Build history of the part. All positions in model axes, mm. A direction names the side the tool comes from. Round coordinates to 2 decimals unless told otherwise and drop trailing zeros. Order: outer loops, then holes, each group sorted by start corner. A loop starts at its lowest first (then second) coordinate and runs counter-clockwise, first axis right, second up. Notation, with made-up numbers: (81.5, 42.25) -> (126.5, 42.25) arc R20 cw to (126.5, 46.25) -> close; hole circle Ø7 at (5.25, 54.25). An arc over 180 degrees is marked (long way). Use a Markdown table: item, result. Add a question column.
Item 1: Pin check, flat tips, straight feed: pin 1 (10 mm diameter, centred on x = 21, z = 15, fed in from +Y); pin 2 (10 mm diameter, centred on x = 20.5, z = 15, fed in from -Y); pin 3 (3.5 mm diameter, centred on y = 40.5, z = 17, fed in from -X). Stop position of each tip, or through.
Item 2: Slice it at B-B, the plane x = 28.5. Give the cut face in (y, z), plus the area to 3 significant figures.
Item 3: Two-plate mould, pull along X, no slides. Class faces 6 (the face through (63.62, 37.564, 17.742)), 7 (the face through (20, 16, 8)), 8 (the face through (64.611, 10.115, 9.874)): released by +X, released by -X, zero draft, split by the parting line, or undercut.
Item 4: 3-axis set-ups, long thin cutter, end or side, ignore diameter. For faces 1 (the face through (65, 29.9, 10)), 2 (the face through (40.377, 17, 10)), 3 (the face through (20, 10, 4)), 4 (the face through (67.8, 55, 18)), 5 (the face through (55, 52, 10)): which of +Z, -Z, +X, -X, +Y, -Y reach the whole face in a straight line?
Item 5: Slice it at C-C, the plane z = 9.5. State how many separate pieces and enclosed holes the cut face has, plus the area to 3 significant figures.
Item 6: Slice it at A-A, the plane x = 5. Give the cut face in (y, z).
Item 7: Probe L1, parallel to X at y = 6.75, z = 10; L2, parallel to X at y = 6.5, z = 10; L3, parallel to X at y = 55, z = 3. List the from-to ranges inside material, lowest first.
from build123d import *

# Parameters (mm, degrees)
SKETCH_13_R          = 1.55
EXTRUDE_6_DEPTH      = 20
SKETCH_15_R          = 6.1
CUT_EXTRUDE_4_DEPTH  = 40.1
SKETCH_16_R          = 1.55
CUT_EXTRUDE_5_DEPTH  = 93.330926639
CUT_EXTRUDE_7_DEPTH  = 105.522724888
EXTRUDE_8_DEPTH      = 20
CUT_EXTRUDE_8_DEPTH  = 4
CUT_EXTRUDE_9_DEPTH  = 5
SKETCH_29_W          = 20
SKETCH_29_H          = 20
SKETCH_29_W_2        = 12
SKETCH_29_H_2        = 12
CUT_EXTRUDE_11_DEPTH = 40.376839
CHAMFER_7_SIZE       = 1


with BuildPart() as part:
    # 草图13 → 凸台-拉伸6 (new body)
    with BuildSketch(Plane.XY):
        Polygon((0, 0), (45, 0), (75, 0), (75, 70), (55, 70), (55, 20), (45, 20), (0, 20), align=None)
        with Locations((65, 40)):
            Circle(SKETCH_13_R, mode=Mode.SUBTRACT)
        with Locations((65, 55)):
            Circle(SKETCH_13_R, mode=Mode.SUBTRACT)
    extrude(amount=EXTRUDE_6_DEPTH)

    # 草图15 → 切除-拉伸4 (cut)
    with BuildSketch(Plane(origin=(0, 70, 0), x_dir=(1, 0, 0), z_dir=(0, 1, 0))):
        with Locations(Location((65, -10, 0), (0, 0, 270))):
            Circle(SKETCH_15_R)
    extrude(amount=-CUT_EXTRUDE_4_DEPTH, mode=Mode.SUBTRACT)

    # 草图16 → 切除-拉伸5 (cut, through all)
    with BuildSketch(Plane(origin=(0, 20, 0), x_dir=(1, 0, 0), z_dir=(0, 1, 0))):
        with Locations(Location((5, -10, 0), (0, 0, 270))):
            Circle(SKETCH_16_R)
        with Locations(Location((20, -10, 0), (0, 0, 270))):
            Circle(SKETCH_16_R)
        with Locations(Location((35, -10, 0), (0, 0, 270))):
            Circle(SKETCH_16_R)
    extrude(amount=-CUT_EXTRUDE_5_DEPTH, mode=Mode.SUBTRACT)

    # 草图24 → 切除-拉伸7 (cut, through all)
    with BuildSketch(Plane(origin=(0, 0, 0), x_dir=(-1, 0, 0), z_dir=(0, 0, -1))):
        with BuildLine():
            Line((-75, 35), (-75, 0))
            Line((-75, 0), (-40, 0))
            ThreePointArc((-40, 0), (-64.748737342, 10.251262658), (-75, 35))
        make_face()
    extrude(amount=-CUT_EXTRUDE_7_DEPTH, mode=Mode.SUBTRACT)

    # 草图25 → 凸台-拉伸8 (add)
    with BuildSketch(Plane(origin=(0, 0, 0), x_dir=(-1, 0, 0), z_dir=(0, 0, -1))):
        with BuildLine():
            Line((-55, 34.995265669), (-55, 20))
            Line((-55, 20), (-40.376838854, 20))
            ThreePointArc((-40.376838854, 20), (-50.739007934, 24.522744072), (-55, 34.995265669))
        make_face()
    extrude(amount=-EXTRUDE_8_DEPTH)

    # 草图26 → 切除-拉伸8 (cut)
    with BuildSketch(Plane.XZ):
        Polygon((4.044652328, 6.911206682), (7.197299644, 7.628247988), (8.152647316, 10.717041306), (5.955347672, 13.088793318), (2.802700356, 12.371752012), (1.847352684, 9.282958694), align=None)
        Polygon((19.044652328, 6.911206682), (22.197299644, 7.628247988), (23.152647316, 10.717041306), (20.955347672, 13.088793318), (17.802700356, 12.371752012), (16.847352684, 9.282958694), align=None)
        Polygon((34.044652328, 6.911206682), (37.197299644, 7.628247988), (38.152647316, 10.717041306), (35.955347672, 13.088793318), (32.802700356, 12.371752012), (31.847352684, 9.282958694), align=None)
    extrude(amount=-CUT_EXTRUDE_8_DEPTH, mode=Mode.SUBTRACT)

    # 草图27 → 切除-拉伸9 (cut)
    with BuildSketch(Plane(origin=(0, 0, 20), x_dir=(-1, 0, 0), z_dir=(0, 0, -1))):
        Polygon((-65, 36.766838493), (-62.2, 38.383419246), (-62.2, 41.616580754), (-65, 43.233161507), (-67.8, 41.616580754), (-67.8, 38.383419246), align=None)
        Polygon((-65, 51.766838493), (-62.2, 53.383419246), (-62.2, 56.616580754), (-65, 58.233161507), (-67.8, 56.616580754), (-67.8, 53.383419246), align=None)
    extrude(amount=CUT_EXTRUDE_9_DEPTH, mode=Mode.SUBTRACT)

    # 草图29 → 切除-拉伸11 (cut)
    with BuildSketch(Plane.ZY):
        with Locations((10, 10)):
            Rectangle(SKETCH_29_W, SKETCH_29_H)
        with Locations((10, 10)):
            Rectangle(SKETCH_29_W_2, SKETCH_29_H_2, mode=Mode.SUBTRACT)
    extrude(amount=-CUT_EXTRUDE_11_DEPTH, mode=Mode.SUBTRACT)

    # 倒角7
    chamfer_7_edges = [part.edges().sort_by_distance(p)[0] for p in [
        (55, 70, 10),
        (75, 70, 10),
        (65, 70, 20),
        (64.881613342, 10.384855932, 0),
        (64.881613342, 10.384855932, 20),
        (0, 16, 10),
        (20.1884195, 16, 16),
        (0, 4, 10),
        (20.1884195, 4, 4),
        (0, 10, 16),
        (20.1884195, 4, 16),
        (0, 10, 4),
        (20.1884195, 16, 4),
        (55, 52.497632834, 20),
        (65, 70, 3.9),
        (75, 52.5, 0),
        (75, 52.5, 20),
        (50.739007934, 24.522744072, 0),
        (50.739007934, 24.522744072, 20),
        (55, 52.497632834, 0),
        (65, 70, 0),
    ]]
    chamfer(chamfer_7_edges, length=CHAMFER_7_SIZE)


solid = part.part
Check sheet entries:
| question | item | result |
|---|---|---|
| 1 | pin 1 | y = 16 |
| 1 | pin 2 | y = 4 |
| 1 | pin 3 | x = 55 |
| 2 | outline | (4, 5) -> (5, 4) -> (15, 4) -> (16, 5) -> (16, 15) -> (15, 16) -> (5, 16) -> (4, 15) -> close |
| 2 | area | 142 mm2 |
| 3 | face 6 | undercut |
| 3 | face 7 | zero draft |
| 3 | face 8 | released by +X |
| 4 | face 1 | +Y |
| 4 | face 2 | -X |
| 4 | face 3 | -Z, -X, +Y, -Y |
| 4 | face 4 | +Z |
| 4 | face 5 | +Z, -Z, -X, +Y |
| 5 | separate pieces | 4 |
| 5 | enclosed holes | 0 |
| 5 | area | 1,370 mm2 |
| 6 | outline | (4, 5) -> (5, 4) -> (15, 4) -> (16, 5) -> (16, 8.45) -> (4, 8.45) -> close; (4, 11.55) -> (16, 11.55) -> (16, 15) -> (15, 16) -> (5, 16) -> (4, 15) -> close |
| 7 | L1 | 0 to 3.45, 6.55 to 18.45, 21.55 to 33.45, 36.55 to 60.66 |
| 7 | L2 | 0 to 3.45, 6.55 to 18.45, 21.55 to 33.45, 36.55 to 60.32 |
| 7 | L3 | 55 to 63.45, 66.55 to 75 |
